```python
from build123d import *

# Parameters (mm, degrees)
F1_DEPTH = 8.6
F2_R     = 12
F3_R     = 21.8
F4_T     = -1.6
F6_DEPTH = 2
F7_SIZE  = 0.99999
F8_W     = 40
F8_H     = 2
F9_DEPTH = 30


# Not quite as in the source:
# - a fillet or chamfer is up to 0.001 mm smaller than in the source, because OpenCascade refuses the exact size


with BuildPart() as f1:
    # F0 (on Top) → F1 (new body)
    with BuildSketch(Plane.XY):
        Polygon((0, 0), (0, 180), (-10.2, 180), (-10.2, 10.2), (-100, 10.2), (-100, 0), align=None)
    extrude(amount=F1_DEPTH)

    # F2
    f2_edges = [f1.edges().sort_by_distance(p)[0] for p in [
        (-10.2, 10.2, 4.3),
    ]]
    fillet(f2_edges, radius=F2_R)

    # F3
    f3_edges = [f1.edges().sort_by_distance(p)[0] for p in [
        (0, 0, 4.3),
    ]]
    fillet(f3_edges, radius=F3_R)

    # F4
    f4_openings = [f1.faces().sort_by_distance(p)[0] for p in [
        (-100, 5.1, 4.3),
        (-2.059126, 100.9, 8.6),
        (-5.1, 180, 4.3),
    ]]
    offset(amount=F4_T, openings=f4_openings)

    # F5 (on face) → F6 (join)
    with BuildSketch(Plane.XY.offset(8.6)):
        with BuildLine():
            ThreePointArc((-22.2, 7.6), (-11.8762409947, 11.8762409947), (-7.6, 22.2))
            Line((-7.6, 22.2), (-7.6, 180))
            Line((-7.6, 180), (-10.2, 180))
            Line((-10.2, 180), (-10.2, 22.2))
            ThreePointArc((-10.2, 22.2), (-13.7147186258, 13.7147186258), (-22.2, 10.2))
            Line((-22.2, 10.2), (-100, 10.2))
            Line((-100, 10.2), (-100, 7.6))
            Line((-100, 7.6), (-22.2, 7.6))
        make_face()
        with BuildLine():
            Line((0, 21.8), (0, 180))
            Line((0, 180), (-2.6, 180))
            Line((-2.6, 180), (-2.6, 21.8))
            ThreePointArc((-2.6, 21.8), (-8.2235498012, 8.2235498012), (-21.8, 2.6))
            Line((-21.8, 2.6), (-100, 2.6))
            Line((-100, 2.6), (-100, 0))
            Line((-100, 0), (-21.8, 0))
            ThreePointArc((-21.8, 0), (-6.3850721701, 6.3850721701), (0, 21.8))
        make_face()
    extrude(amount=-F6_DEPTH)

    # F7 (size 1 in the source; OpenCascade refuses exactly that, so slightly less here)
    f7_edges = [f1.edges().sort_by_distance(p)[0] for p in [
        (-61.1, 7.6, 6.6),
        (-60.9, 2.6, 6.6),
    ]]
    chamfer(f7_edges, length=F7_SIZE)

    # F8 (on Top) → F9 (join)
    with BuildSketch(Plane.XY):
        with Locations((-50, 10)):
            Rectangle(F8_W, F8_H)
    extrude(amount=F9_DEPTH)


solid = f1.part
```
Design review of the part built by this model. Coordinates are the model's own, in mm. A direction names the side the tool comes from. Give positions to 0.01 mm unless a question says otherwise; leave off trailing zeros. Write each loop counter-clockwise with the first axis right and the second up, starting at its lowest first coordinate (ties: lowest second). Pieces come first, ordered by that corner, then holes.
(1) Add section C-C (z = 11.75). Give the boundary of the cut face in (x, y), and give its area (3 significant figures).
Checked values:
outline: (-70, 9) - (-30, 9) - (-30, 11) - (-70, 11) - close
area: 80.0 mm2
(2) Tool access review of faces 5 (the face through (-26, 10.2, 4)), 6 (the face through (-11.99, 11.763, 8.107)), 7 (the face through (-7.36, 7.674, 4.135)), 8 (the face through (-85, 10.2, 4)), 9 (the face through (-61, 0, 4)): name each direction out of +Z, -Z, +X, -X, +Y, -Y from which nothing blocks a thin tool from reaching the whole face with its end or side.
Checked values:
face 5: +Z, -Z, +Y
face 6: +Z
face 7: none
face 8: +Z, -Z, -X, +Y
face 9: +Z, -Z, +X, -X, -Y
(3) Clearance check with flat-ended pins moving along their axes: pin 1 Ø1.6 at (y, z) = (10, 19) entering from -X; pin 2 Ø9.5 at (x, z) = (-86.5, 5) entering from +Y; pin 3 Ø4 at (y, z) = (129.5, 5) entering from -X. State where each tip first meets the part, or that it passes through.
Checked values:
pin 1: stops at x = -70
pin 2: stops at y = 10.2
pin 3: stops at x = -10.2
(4) Mouldability with a two-part tool opening along Z and no side actions: class faces 1 (the face through (-2, 90, 8.6)), 2 (the face through (-12.568, 12.354, 6.774)), 3 (the face through (-61, 1.6, 4)), 4 (the face through (-6.217, 6.555, 4.36)) as +Z half, -Z half, draft (parallel to the pull), parting line (faces both ways), or undercut.
Checked values:
face 1: +Z half
face 2: undercut
face 3: undercut
face 4: draft
(5) Wall thickness on line 1 along X through (y, z) = (145, 4.5); line 2 along Y through (x, z) = (-41, 3.5); line 3 along Y through (x, z) = (-39.5, 26.75): over which ranges is each line inside the solid? List them lowest first.
Checked values:
line 1: x = -10.2 to -8.6, -1.6 to 0
line 2: y = 0 to 1.6, 8.6 to 11
line 3: y = 9 to 11
